Read the model definition and answer for the solid it produces. Units are mm, in the model's axes. Face numbers are marked on the shaded views. Coordinates: 2 decimals unless noted, no trailing zeros. Loops run counter-clockwise (first coordinate to the right, second up) from the corner with the lowest first, then second, coordinate; pieces in that order, holes last.
Q1. Section D-D (x = -24) is taken. Give the vertices of the cut face in (y, z), then the cut area to 3 significant figures.
Q2. Flat-ended cylindrical pins translate along their axes: P1, Ø4, axis at y = 4.5, z = 3.5, coming from the +X side; P2, Ø4, axis at y = 32, z = 6.5, coming from the -X side; P3, Ø1.5, axis at y = -3.5, z = 1, coming from the +X side. Find the tip coordinate at first contact, or state that the pin passes through.
Q3. Section C-C (y = 39) is taken. Give the vertices of the cut face in (x, z), then the cut area to 3 significant figures.
Q4. The mould has two halves that part along Y. Classify the marked faces 1, 2 and 3: pulls with the +Y half, pulls with the -Y half, needs draft (parallel to the pull), parting line crosses it, or undercut.
Q5. Straight lines are drawn through the part: line 1 (X direction, y = -11, z = 0); line 2 (X direction, y = 44, z = -7.5); line 3 (X direction, y = 8, z = 2). For each, find the intervals that lie inside material, in ascending order.
Q6. Section A-A (x = 41) is taken. Give the vertices of the cut face in (y, z), then the cut area to 3 significant figures.
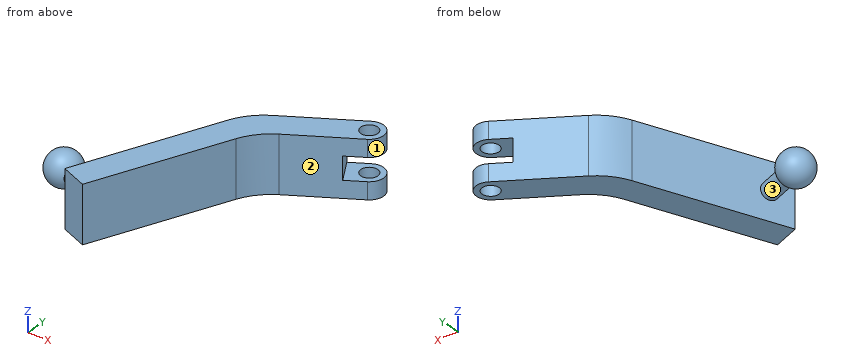
from build123d import *

# Parameters (mm, degrees)
BOSS_EXTRU_1_DEPTH      = 10
BOSS_EXTRU_1_DEPTH_BACK = 10
ESQUISSE2_W             = 16.778324123
ESQUISSE2_H             = 8
ENL_V_MAT_EXTRU_2_DEPTH = 77.675205123
ESQUISSE3_R             = 3
ENL_V_MAT_EXTRU_3_DEPTH = 74.486360502
ESQUISSE4_R             = 3
BOSS_EXTRU_2_DEPTH      = 10
CONG_2_R                = 5


with BuildPart() as part:
    # Esquisse1 → Boss.-Extru.1 (new, two sides: drawn at the far end of the back side and taken through both)
    with BuildSketch(Plane.XY.offset(-BOSS_EXTRU_1_DEPTH_BACK)):
        with BuildLine():
            Line((42.458304448, 52.329533504), (13.73470128, 35.295768835))
            ThreePointArc((13.73470128, 35.295768835), (8.854424282, 31.228601734), (5.495862123, 25.836105835))
            Line((5.495862123, 25.836105835), (-15.175609455, -23.394635688))
            Line((-15.175609455, -23.394635688), (-5.955424705, -27.266094479))
            Line((-5.955424705, -27.266094479), (13.437406292, 18.919463554))
            ThreePointArc((13.437406292, 18.919463554), (16.795968451, 24.311959453), (21.676245449, 28.379126554))
            Line((21.676245449, 28.379126554), (47.55906962, 43.728243213))
            Line((47.55906962, 43.728243213), (42.458304448, 52.329533504))
        make_face()
    extrude(amount=BOSS_EXTRU_1_DEPTH + BOSS_EXTRU_1_DEPTH_BACK)

    # Esquisse2 → Enlèv. mat.-Extru.2 (cut, through all)
    with BuildSketch(Plane(origin=(-11.911901978, 20.08673667, 0), x_dir=(0.8601290290322577, 0.5100765172168049, 0), z_dir=(-0.5100765172168049, 0.8601290290322577, 0))):
        with Locations((59.600848438, 0)):
            Rectangle(ESQUISSE2_W, ESQUISSE2_H)
    extrude(amount=-ENL_V_MAT_EXTRU_2_DEPTH, mode=Mode.SUBTRACT)

    # Esquisse3 → Enlèv. mat.-Extru.3 (cut, through all)
    with BuildSketch(Plane.XY.offset(10)):
        with Locations((40.705018812, 45.476713018)):
            Circle(ESQUISSE3_R)
    extrude(amount=-ENL_V_MAT_EXTRU_3_DEPTH, mode=Mode.SUBTRACT)

    # Esquisse4 → Boss.-Extru.2 (add)
    with BuildSketch(Plane(origin=(-4.550212337, 1.910586396, 0), x_dir=(0, 0, 1), z_dir=(-0.9220184750588774, 0.38714587903024655, 0))):
        with Locations(Location((0, -19.124935546, 0), (0, 0, 270))):
            Circle(ESQUISSE4_R)
    extrude(amount=BOSS_EXTRU_2_DEPTH)

    # Esquisse5 → Révolution1 (revolve)
    with BuildSketch(Plane.XY):
        with BuildLine():
            Line((-20.095687486, -12.304496338), (-31.159909187, -7.658745789))
            ThreePointArc((-31.159909187, -7.658745789), (-23.304923062, -4.449510213), (-20.095687486, -12.304496338))
        make_face()
    revolve(axis=Axis((-21.174537071, -11.851498722, 0), (-0.9220184750588776, 0.3871458790302464, 0)))

    # Congé2
    cong_2_edges = [part.edges().sort_by_distance(p)[0] for p in [
        (47.55906962, 43.728243213, 7),
        (42.458304448, 52.329533504, 7),
        (42.458304448, 52.329533504, -7),
        (47.55906962, 43.728243213, -7),
    ]]
    fillet(cong_2_edges, radius=CONG_2_R - 0.0001)  # a hair under: the kernel refuses the full size


solid = part.part
Numbers:
1. outline: circle Ø11.55 at (-9.98, 0)
1. area: 105 mm2
2. P1: stops at x = 8.22
2. P2: stops at x = 7.87
2. P3: stops at x = 4.34
3. outline: (19.98, -10) - (39.59, -10) - (39.59, -4) - (36.41, -4) - (36.41, 4) - (39.59, 4) - (39.59, 10) - (19.98, 10) - close
3. area: 367 mm2
4. face 1: parting line crosses it
4. face 2: pulls with the -Y half
4. face 3: undercut
5. line 1: x = -31.54 to -15.45, -9.97 to 0.87
5. line 2: x = 28.41 to 38.09, 43.32 to 45.48
5. line 3: x = -1.99 to 8.85
6. outline: (39.84, -10) - (42.49, -10) - (42.49, -4) - (39.84, -4) - close; (39.84, 4) - (42.49, 4) - (42.49, 10) - (39.84, 10) - close; (48.46, -10) - (50.47, -10) - (50.47, -4) - (48.46, -4) - close; (48.46, 4) - (50.47, 4) - (50.47, 10) - (48.46, 10) - close
6. area: 55.9 mm2
